For this review, take the finished solid that the model builds, in its own axes (mm). Give positions to 0.01 mm unless a question says otherwise; leave off trailing zeros. Write each loop counter-clockwise with the first axis right and the second up, starting at its lowest first coordinate (ties: lowest second). Pieces come first, ordered by that corner, then holes.
Q1. We need section C-C (x = -522). Write out the cut boundary in (y, z) (3 decimals), then the cut area to 3 significant figures.
Q2. Insertion check: P1, Ø2.5, axis at x = -240.5, y = 24.5, coming from the -Z side. The pin has a flat end and moves straight along its axis. Give the tip position at first contact, or say it passes through.
Q3. For line 1 (Z direction, x = -400.5, y = 17.5) (3 decimals); line 2 (Z direction, x = -57, y = 4.75) (3 decimals), list the stretches that pass through material, from the lowest coordinate up.
Q4. We need section B-B (z = 8). Write out the cut boundary in (x, y) (3 decimals), then the cut area to 3 significant figures.
Q5. We need section A-A (y = 10.75). Write out the cut boundary in (x, z) (3 decimals), then the cut area to 3 significant figures.
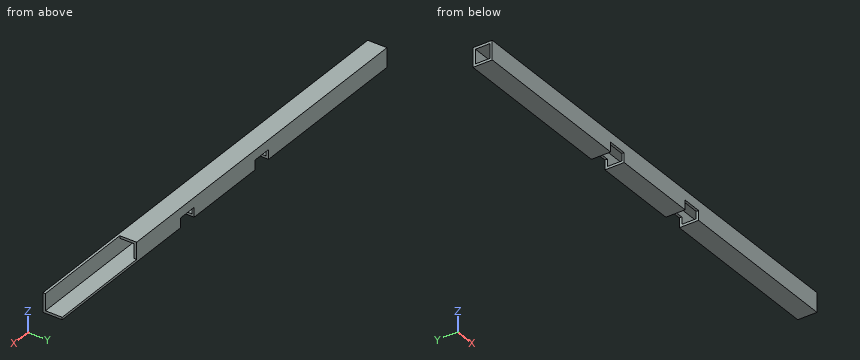
Autodesk Inventor part; units mm, degrees
ref_plane "YZ Plane" through (0, 0, 0) normal (1, 0, 0) x (0, 1, 0)
ref_plane "XZ Plane" through (0, 0, 0) normal (0, 1, 0) x (-1, 0, 0)
ref_plane "XY Plane" through (0, 0, 0) normal (0, 0, 1) x (1, 0, 0)
sketch "Sketch1" plane through (0, 0, 0) normal (0, 0, 1) x (1, 0, 0)
  line L0 (0, 0) -> (-609.6, 0)
  line L1 (-609.6, 0) -> (-609.6, 25.4)
  line L2 (-609.6, 25.4) -> (0, 25.4)
  line L3 (0, 25.4) -> (0, 0)
  dimension "d0" = 25.4
  dimension "d1" = 609.6
extrude "Extrusion1" add sketch "Sketch1" along normal blind 25.4
shell "Shell2" thickness 3.175 removed faces 2 at (-609.6, 8.4667, 16.9333) at (0, 16.9333, 8.4667)
sketch "Sketch3" plane through (0, 0, 25.4) normal (0, 0, 1) x (1, 0, 0)
  line L0 (0, 25.4) -> (-139.7, 25.4)
  line L1 (-139.7, 25.4) -> (-139.7, 3.175)
  line L2 (-139.7, 3.175) -> (0, 3.175)
  line L3 (0, 3.175) -> (0, 25.4)
  dimension "d9" = 22.225
  dimension "d10" = 139.7
extrude "Extrusion3" cut sketch "Sketch3" against normal blind 22.225
sketch "Sketch4" plane through (-609.6, 0, 0) normal (0, -1, 0) x (1, 0, 0)
  line L0 (361.95, 0) -> (387.35, 0)
  line L1 (387.35, 0) -> (387.35, 12.7)
  line L2 (387.35, 12.7) -> (361.95, 12.7)
  line L3 (361.95, 12.7) -> (361.95, 0)
  line L4 (222.25, 0) -> (247.65, 0)
  line L5 (247.65, 0) -> (247.65, 12.7)
  line L6 (247.65, 12.7) -> (222.25, 12.7)
  line L7 (222.25, 12.7) -> (222.25, 0)
  line L8 (222.25, 0) -> (0, 0) construction
  line L9 (387.35, 0) -> (609.6, 0) construction
  dimension "d13" = 12.7
  dimension "d14" = 25.4
  dimension "d18" = 114.3
extrude "Extrusion4" cut sketch "Sketch4" against normal through all
properties part number "Shovel_CrossFrame" material "Aluminum-6061"
Computed:
1. outline: (0, 0) - (25.4, 0) - (25.4, 25.4) - (0, 25.4) - close; hole (3.175, 3.175) - (22.225, 3.175) - (22.225, 22.225) - (3.175, 22.225) - close
1. area: 282 mm2
2. P1: stops at z = 12.7
3. line 1: z = 0 to 3.175, 22.225 to 25.4
3. line 2: z = 0 to 3.175
4. outline: (-609.6, 0) - (-387.35, 0) - (-387.35, 3.175) - (-609.6, 3.175) - close; (-609.6, 22.225) - (-387.35, 22.225) - (-387.35, 25.4) - (-609.6, 25.4) - close; (-361.95, 0) - (-247.65, 0) - (-247.65, 3.175) - (-361.95, 3.175) - close; (-361.95, 22.225) - (-247.65, 22.225) - (-247.65, 25.4) - (-361.95, 25.4) - close; (-222.25, 0) - (0, 0) - (0, 3.175) - (-222.25, 3.175) - close; (-222.25, 22.225) - (-139.7, 22.225) - (-139.7, 25.4) - (-222.25, 25.4) - close
4. area: 3,100 mm2
5. outline: (-609.6, 0) - (-387.35, 0) - (-387.35, 3.175) - (-609.6, 3.175) - close; (-609.6, 22.225) - (-139.7, 22.225) - (-139.7, 25.4) - (-609.6, 25.4) - close; (-361.95, 0) - (-247.65, 0) - (-247.65, 3.175) - (-361.95, 3.175) - close; (-222.25, 0) - (0, 0) - (0, 3.175) - (-222.25, 3.175) - close
5. area: 3,270 mm2
